Geometry check sheet. Reference: the model listing, model coordinates, mm. Coordinates: 2 decimals unless noted, no trailing zeros. Loops run counter-clockwise (first coordinate to the right, second up) from the corner with the lowest first, then second, coordinate; pieces in that order, holes last.
from build123d import *

# Parameters (mm, degrees)
SKETCH1_R           = 3.302
BOSS_EXTRUDE1_DEPTH = 5
SKETCH2_R           = 1.05
CUT_EXTRUDE2_DEPTH  = 108.879006299


with BuildPart() as part:
    # Sketch1 → Boss-Extrude1 (new body)
    with BuildSketch(Plane(origin=(0, 0, 0), x_dir=(1, 0, 0), z_dir=(0, 1, 0))):
        with BuildLine():
            Line((-69.85, 76.2), (69.85, 76.2))
            ThreePointArc((69.85, 76.2), (74.340128061, 74.340128061), (76.2, 69.85))
            Line((76.2, 69.85), (76.2, -69.85))
            ThreePointArc((76.2, -69.85), (74.340128061, -74.340128061), (69.85, -76.2))
            Line((69.85, -76.2), (-69.85, -76.2))
            ThreePointArc((-69.85, -76.2), (-74.340128061, -74.340128061), (-76.2, -69.85))
            Line((-76.2, -69.85), (-76.2, 69.85))
            ThreePointArc((-76.2, 69.85), (-74.340128061, 74.340128061), (-69.85, 76.2))
        make_face()
        with Locations(Location((63.5, 63.5, 0), (0, 0, 270))):
            Circle(SKETCH1_R, mode=Mode.SUBTRACT)
        with Locations(Location((63.5, -63.5, 0), (0, 0, 90))):
            Circle(SKETCH1_R, mode=Mode.SUBTRACT)
        with Locations(Location((-63.5, -63.5, 0), (0, 0, 270))):
            Circle(SKETCH1_R, mode=Mode.SUBTRACT)
        with Locations(Location((-63.5, 63.5, 0), (0, 0, 90))):
            Circle(SKETCH1_R, mode=Mode.SUBTRACT)
        with Locations(Location((0, 0, 0), (0, 0, 270))):
            Circle(SKETCH1_R, mode=Mode.SUBTRACT)
    extrude(amount=BOSS_EXTRUDE1_DEPTH)

    # Sketch2 → Cut-Extrude2 (cut, through all)
    with BuildSketch(Plane(origin=(0, 0, 0), x_dir=(1, 0, 0), z_dir=(0, 1, 0))):
        with Locations(Location((-42.055175811, -29.786873157, 0), (0, 0, 270))):
            Circle(SKETCH2_R)
        with Locations(Location((-22.079409243, -49.762639726, 0), (0, 0, 270))):
            Circle(SKETCH2_R)
        with Locations(Location((22.079409243, -49.762639726, 0), (0, 0, 90))):
            Circle(SKETCH2_R)
        with Locations(Location((42.055175811, -29.786873157, 0), (0, 0, 90))):
            Circle(SKETCH2_R)
        with BuildLine():
            Line((-33.693638124, -42.673894245), (-34.428769513, -41.938762855))
            ThreePointArc((-34.428769513, -41.938762855), (-40.305086528, -31.536962441), (-29.903286113, -37.413279456))
            Line((-29.903286113, -37.413279456), (-29.168154724, -38.148410845))
            ThreePointArc((-29.168154724, -38.148410845), (-29.168154724, -42.673894245), (-33.693638124, -42.673894245))
        make_face()
        with BuildLine():
            Line((33.693638124, -42.673894245), (34.428769513, -41.938762855))
            ThreePointArc((34.428769513, -41.938762855), (40.305086528, -31.536962441), (29.903286113, -37.413279456))
            Line((29.903286113, -37.413279456), (29.168154724, -38.148410845))
            ThreePointArc((29.168154724, -38.148410845), (29.168154724, -42.673894245), (33.693638124, -42.673894245))
        make_face()
    extrude(amount=CUT_EXTRUDE2_DEPTH, mode=Mode.SUBTRACT)


solid = part.part
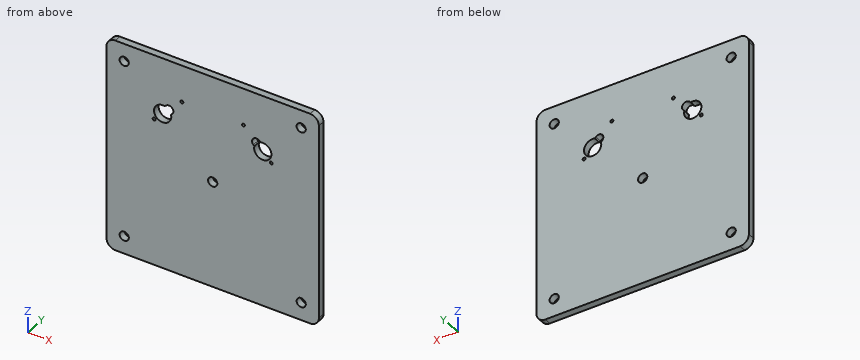
(1) Sectioned sample at B-B on z = 0. Record the cut outline in (x, y), and give its area (3 significant figures).
Findings:
outline: (-76.2, 0) - (-3.3, 0) - (-3.3, 5) - (-76.2, 5) - close; (3.3, 0) - (76.2, 0) - (76.2, 5) - (3.3, 5) - close
area: 729 mm2
(2) Sectioned sample at C-C on x = 0. Record the cut outline in (y, z), and give its area (3 significant figures).
Findings:
outline: (0, -76.2) - (5, -76.2) - (5, -3.3) - (0, -3.3) - close; (0, 3.3) - (5, 3.3) - (5, 76.2) - (0, 76.2) - close
area: 729 mm2
(3) Scan lines: L1, parallel to X at y = 3.7, z = -63.5; L2, parallel to Z at x = 62.5, y = 1.5; L3, parallel to X at y = 3.8, z = 31. Record each from-to range of solid material in increasing order.
Findings:
L1: x = -76.2 to -66.8, -60.2 to 60.2, 66.8 to 76.2
L2: z = -76.2 to -66.65, -60.35 to 60.35, 66.65 to 76.2
L3: x = -76.2 to -39.69, -32.15 to 32.15, 39.69 to 76.2
(4) Sectioned sample at D-D on z = 63.5. Record the cut outline in (x, y), and give its area (3 significant figures).
Findings:
outline: (-76.2, 0) - (-66.8, 0) - (-66.8, 5) - (-76.2, 5) - close; (-60.2, 0) - (60.2, 0) - (60.2, 5) - (-60.2, 5) - close; (66.8, 0) - (76.2, 0) - (76.2, 5) - (66.8, 5) - close
area: 696 mm2
(5) Sectioned sample at A-A on x = -63.5. Record the cut outline in (y, z), and give its area (3 significant figures).
Findings:
outline: (0, -76.2) - (5, -76.2) - (5, -66.8) - (0, -66.8) - close; (0, -60.2) - (5, -60.2) - (5, 60.2) - (0, 60.2) - close; (0, 66.8) - (5, 66.8) - (5, 76.2) - (0, 76.2) - close
area: 696 mm2
